```python
from build123d import *

# Parameters (mm, degrees)
F1_DEPTH = 100
F3_DEPTH = 25
F4_R     = 10


with BuildPart() as f1:
    # F0 (on Front) → F1 (new body)
    with BuildSketch(Plane.XZ):
        Polygon((15, 0), (0, 0), (0, -20), (50, -20), (50, -70), (65, -70), (65, -10), (15, -10), align=None)
    extrude(amount=F1_DEPTH)

    # F2 (on face) → F3 (cut)
    with BuildSketch(Plane.YZ.offset(65)):
        with BuildLine():
            Line((-20, -32.5), (-80, -32.5))
            ThreePointArc((-80, -32.5), (-87.5, -40), (-80, -47.5))
            Line((-80, -47.5), (-20, -47.5))
            ThreePointArc((-20, -47.5), (-12.5, -40), (-20, -32.5))
        make_face()
    extrude(amount=-F3_DEPTH, mode=Mode.SUBTRACT)

    # F4
    f4_edges = [f1.edges().sort_by_distance(p)[0] for p in [
        (57.5, -100, -70),
        (57.5, 0, -70),
    ]]
    fillet(f4_edges, radius=F4_R)


solid = f1.part
```
Input: part model. Units: mm. Frame: model coordinates. A direction names the side the tool comes from. Round coordinates to 2 decimals unless told otherwise and drop trailing zeros. Loops run counter-clockwise (first coordinate to the right, second up) from the corner with the lowest first, then second, coordinate; pieces in that order, holes last. Notation, with made-up numbers: M 20,39 L 26,39 A16 cw 26,59 Z; hole C 81,69.25 d10. An arc over 180 degrees is marked long. Answer in a Markdown table with one row per item. Add a question column.
1. Section B-B (y = -47). Output: boundary loops of the cut face in (x, z).
2. Ray query, probe 1 along Z at (x, y) = (13, -61.5); probe 2 along X at (y, z) = (-90.5, -41.5); probe 3 along Z at (x, y) = (25, -13.5). Return the intervals inside material, ascending.
3. Section A-A (x = 58). Output: boundary loops of the cut face in (y, z), and give its area (3 significant figures).
4. Section C-C (z = -40). Output: boundary loops of the cut face in (x, y).
5. Mould query, pull axis Y, two halves, no side actions, for faces 1 (the face through (58, -50, -32.5)), 2 (the face through (37, 0, -19)), 3 (the face through (37, -100, -19)). Classes: released by +Y, released by -Y, zero draft, split by the parting line, or undercut.
6. Set-up query: faces 4 (the face through (15, -49, -5)), 5 (the face through (25, -49, -20)), 6 (the face through (57.6, -12.5, -40.16)). Return all of +Z, -Z, +X, -X, +Y, -Y with unobstructed straight access to the full face (end or side cutting, diameter ignored); none if empty.
7. Contact query for flat-ended pins moving along their axis: pin 1 (25 mm diameter, centred on y = -27, z = -37, fed in from -X); pin 2 (3 mm diameter, centred on y = -54, z = -5.5, fed in from +X); pin 3 (12 mm diameter, centred on x = 54.5, y = -61.5, fed in from +Z); pin 4 (10 mm diameter, centred on y = -78, z = -24, fed in from -X). Output: stop coordinate, or through.
8. Section D-D (y = -91.5). Output: boundary loops of the cut face in (x, z), and give its area (3 significant figures).
Values follow:
| question | item | result |
|---|---|---|
| 1 | outline | M 0,-20 L 50,-20 L 50,-32.5 L 65,-32.5 L 65,-10 L 15,-10 L 15,0 L 0,0 Z; M 50,-70 L 65,-70 L 65,-47.5 L 50,-47.5 Z |
| 2 | probe 1 | -20 to 0 |
| 2 | probe 2 | 50 to 65 |
| 2 | probe 3 | -20 to -10 |
| 3 | outline | M -100,-60 A10 ccw -90,-70 L -10,-70 A10 ccw 0,-60 L 0,-10 L -100,-10 Z; hole M -80,-47.5 L -20,-47.5 A7.5 ccw -20,-32.5 L -80,-32.5 A7.5 ccw Z |
| 3 | area | 4,880 mm^2 |
| 4 | outline | M 50,-100 L 65,-100 L 65,-87.5 L 50,-87.5 Z; M 50,-12.5 L 65,-12.5 L 65,0 L 50,0 Z |
| 5 | face 1 | undercut |
| 5 | face 2 | released by +Y |
| 5 | face 3 | released by -Y |
| 6 | face 4 | +Z, +X, +Y, -Y |
| 6 | face 5 | -Z, -X, +Y, -Y |
| 6 | face 6 | +X, -X |
| 7 | pin 1 | x = 50 |
| 7 | pin 2 | x = 15 |
| 7 | pin 3 | z = -10 |
| 7 | pin 4 | x = 0 |
| 8 | outline | M 0,-20 L 50,-20 L 50,-69.89 L 65,-69.89 L 65,-10 L 15,-10 L 15,0 L 0,0 Z |
| 8 | area | 1,550 mm^2 |
